```python
from build123d import *

# Parameters (mm, degrees)
F1_DEPTH = 70
F2_W     = 5
F2_H     = 35
F3_DEPTH = 70
F6_DEPTH = 38


with BuildPart() as f1:
    # F0 (on Front) → F1 (new body)
    with BuildSketch(Plane.XZ):
        Polygon((-55, 38), (-60, 38), (-60, 0), (-20, 0), (-20, 3), (-55, 3), align=None)
    extrude(amount=F1_DEPTH)


with BuildPart() as f3:
    # F2 (on face) → F3 (new body)
    with BuildSketch(Plane.YZ.offset(-55)):
        with Locations((-2.5, 20.5)):
            Rectangle(F2_W, F2_H)
        Polygon((-40, 0), (0, 0), (0, 3), (-5, 3), (-40, 3), align=None)
    extrude(amount=F3_DEPTH)


with BuildPart() as f1_1:
    add(f1.part)

    # F4: union F3
    add(f3.part)

    # F5 (on face) → F6 (join, through all)
    with BuildSketch(Plane(origin=(0, 0, 0), x_dir=(1, 0, 0), z_dir=(0, 0, -1))):
        Polygon((-60, 5.303301), (-65.303301, 5.303301), (-60, 0), align=None)
        Polygon((-54.696699, 0), (-60, 0), (-54.696699, -5.303301), align=None)
    extrude(amount=-F6_DEPTH)


solid = f1_1.part
```
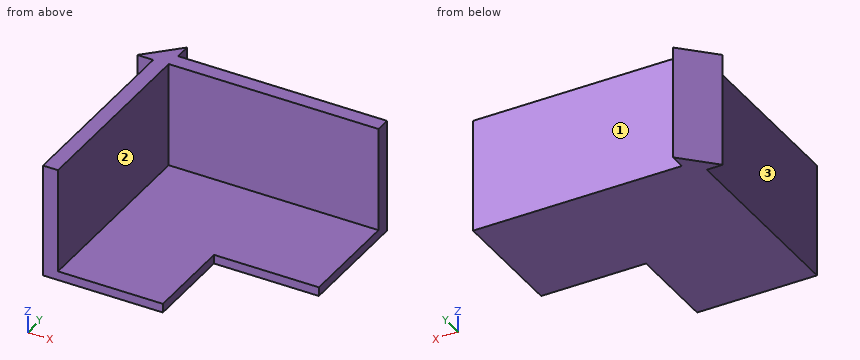
Design review of the part built by this model. Coordinates are the model's own, in mm. Face numbers are marked on the shaded views. A direction names the side the tool comes from. Coordinates: 2 decimals unless noted, no trailing zeros. Order: outer loops, then holes, each group sorted by start corner. A loop starts at its lowest first (then second) coordinate and runs counter-clockwise, first axis right, second up. Notation, with made-up numbers: M 77,20 L 94,20 A13 ccw 94,45 Z; hole C 38.25,-6 d9. An arc over 180 degrees is marked long. Answer as a JSON object with one key per item and string values. Group by question number.
1) Tool access review of the marked faces 1, 2 and 3: name each direction out of +Z, -Z, +X, -X, +Y, -Y from which nothing blocks a thin tool from reaching the whole face with its end or side.
2) Add section B-B, the plane y = -55.5. Write out the cut boundary in (x, z), then the cut area to 3 significant figures.
3) Wall thickness on L1, parallel to X at y = -19.5, z = 4.5; L2, parallel to Y at x = -20, z = 8; L3, parallel to Y at x = -46.5, z = 2: over which ranges is each line inside the solid? List them lowest first.
4) Add section C-C, the plane x = -10. Write out the cut boundary in (y, z), then the cut area to 3 significant figures.
5) For pin 1 (1 mm diameter, centred on x = -17, z = 18, fed in from -Y); pin 2 (1.5 mm diameter, centred on y = -13.5, z = 18.5, fed in from -X); pin 3 (17.5 mm diameter, centred on y = -37, z = 21, fed in from +X), all flat-tipped, find the tip position at first contact; note any pin that passes through.
6) Add section A-A, the plane z = 33.5. Write out the cut boundary in (x, y), then the cut area to 3 significant figures.
Computed values:
{
 "1": {"face 1": "+Z, -Z, +X, +Y", "face 2": "+Z, +X, -Y", "face 3": "+Z, -Z, -X, -Y"},
 "2": {"outline": "M -60,0 L -20,0 L -20,3 L -55,3 L -55,38 L -60,38 Z", "area": "295 mm^2"},
 "3": {"L1": "x = -60 to -55", "L2": "y = -5 to 0", "L3": "y = -70 to 0"},
 "4": {"outline": "M -40,0 L 0,0 L 0,38 L -5,38 L -5,3 L -40,3 Z", "area": "295 mm^2"},
 "5": {"pin 1": "stops at y = -5", "pin 2": "stops at x = -60", "pin 3": "stops at x = -55"},
 "6": {"outline": "M -65.3,-5.3 L -60,-5.3 L -60,-70 L -55,-70 L -55,-5 L 15,-5 L 15,0 L -54.7,0 L -54.7,5.3 Z", "area": "728 mm^2"}
}
